```python
from build123d import *

# Parameters (mm, degrees)
SKETCH1_W           = 100
SKETCH1_H           = 55
BOSS_EXTRUDE1_DEPTH = 3
SKETCH2_W           = 100
SKETCH2_H           = 83
BOSS_EXTRUDE2_DEPTH = 3
BOSS_EXTRUDE3_DEPTH = 3
BOSS_EXTRUDE4_DEPTH = 3
SKETCH5_R           = 13
SKETCH5_R_2         = 2.15
CUT_EXTRUDE1_DEPTH  = 4


with BuildPart() as part:
    # Sketch1 → Boss-Extrude1 (new body)
    with BuildSketch(Plane(origin=(0, 0, 0), x_dir=(1, 0, 0), z_dir=(0, 1, 0))):
        Rectangle(SKETCH1_W, SKETCH1_H)
    extrude(amount=BOSS_EXTRUDE1_DEPTH)

    # Sketch2 → Boss-Extrude2 (add)
    with BuildSketch(Plane.XY.offset(27.5)):
        with Locations((0, -13.5)):
            Rectangle(SKETCH2_W, SKETCH2_H)
    extrude(amount=BOSS_EXTRUDE2_DEPTH)

    # Sketch3 → Boss-Extrude3 (add)
    with BuildSketch(Plane(origin=(50, 0, 0), x_dir=(0, 0, -1), z_dir=(1, 0, 0))):
        Polygon((-27.5, 0), (22.5, 0), (-27.5, -50), align=None)
    extrude(amount=-BOSS_EXTRUDE3_DEPTH)

    # Sketch4 → Boss-Extrude4 (add)
    with BuildSketch(Plane.ZY.offset(50)):
        Polygon((27.5, 0), (27.5, -50), (-22.5, 0), align=None)
    extrude(amount=-BOSS_EXTRUDE4_DEPTH)

    # Sketch5 → Cut-Extrude1 (cut, through all)
    with BuildSketch(Plane(origin=(0, 0, 27.5), x_dir=(-1, 0, 0), z_dir=(0, 0, -1))):
        with Locations((0, -25)):
            Circle(SKETCH5_R)
        with Locations((12.148789351, -12.404091248)):
            Circle(SKETCH5_R_2)
        with Locations((12.595908752, -37.148789351)):
            Circle(SKETCH5_R_2)
        with Locations((-12.148789351, -37.595908752)):
            Circle(SKETCH5_R_2)
        with Locations((-12.595908752, -12.851210649)):
            Circle(SKETCH5_R_2)
    extrude(amount=-CUT_EXTRUDE1_DEPTH, mode=Mode.SUBTRACT)


solid = part.part
```
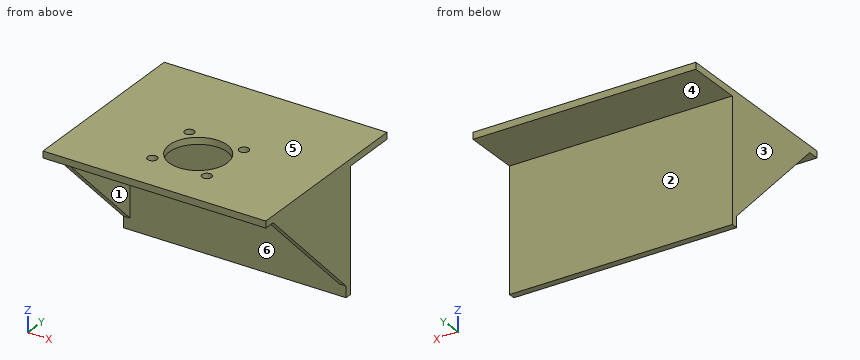
Geometry: final body of the model. Coordinates: model frame, mm. Face numbers are marked on the shaded views. A direction names the side the tool comes from. Round coordinates to 2 decimals unless told otherwise and drop trailing zeros. Order: outer loops, then holes, each group sorted by start corner. A loop starts at its lowest first (then second) coordinate and runs counter-clockwise, first axis right, second up. Notation, with made-up numbers: (78.25, 60) - (128.25, 60) arc R22 cw to (128.25, 79) - close; hole circle Ø5 at (9, -19). An arc over 180 degrees is marked (long way). Write item = value, one per line. Start each with the question number.
Q1. Cut plane C-C on z = 23. Return the cut outline in (x, y), and give its area (3 significant figures).
Q2. Access query for the marked faces 4, 5 and 6. Directions: +Z, -Z, +X, -X, +Y, -Y. A direction counts if a zero-diameter tool reaches every point of the face in a straight line with its end or side. Return the directions, or none.
Q3. Pin query (flat end, axial travel): pin 1 (3 mm diameter, centred on x = 11, z = 5, fed in from -Y); pin 2 (2 mm diameter, centred on x = 29, y = -20.5, fed in from -Z); pin 3 (1 mm diameter, centred on x = 37.5, z = 18, fed in from +Y); pin 4 (25 mm diameter, centred on y = -35.5, z = 3.5, fed in from -X). Return the tip coordinate at first contact, or that it passes through.
Q4. Pull-direction query (X, two-part tool) for the marked faces 1, 2 and 3; classes: +X half, -X half, draft (parallel to the pull), parting line (faces both ways), or undercut.
Q5. Cut plane A-A on x = 0. Return the cut outline in (y, z).
Q6. Ray query, line 1 (Y direction, x = 5, z = -1); line 2 (Z direction, x = 43, y = 7.5); line 3 (X direction, y = -17, z = 11.5). Return the intervals inside material, ascending. Write a range as from..to.
Q7. Cut plane D-D on x = -40. Return the cut outline in (y, z).
Q8. Cut plane B-B on y = -25. Return the cut outline in (x, z).
Outcome:
q1.outline = (-50, -45.5) - (-47, -45.5) - (-47, 0) - (47, 0) - (47, -45.5) - (50, -45.5) - (50, 3) - (-50, 3) - close
q1.area = 573 mm^2
q2.face_4 = -Z, +X, -X, +Y
q2.face_5 = +Z, +X, -X, +Y, -Y
q2.face_6 = -Z, -Y
q3.pin_1 = 0
q3.pin_2 = 27.5
q3.pin_3 = 3
q3.pin_4 = -50
q4.face_1 = undercut
q4.face_2 = draft
q4.face_3 = -X half
q5.outline = (-55, 27.5) - (-38, 27.5) - (-38, 30.5) - (-55, 30.5) - close; (-12, 27.5) - (0, 27.5) - (0, -27.5) - (3, -27.5) - (3, 27.5) - (28, 27.5) - (28, 30.5) - (-12, 30.5) - close
q6.line_1 = 0..3
q6.line_2 = 27.5..30.5
q6.line_3 = -50..-47, 47..50
q7.outline = (-55, 27.5) - (0, 27.5) - (0, -27.5) - (3, -27.5) - (3, 27.5) - (28, 27.5) - (28, 30.5) - (-55, 30.5) - close
q8.outline = (-50, 2.5) - (-47, 2.5) - (-47, 27.5) - (-13, 27.5) - (-13, 30.5) - (-50, 30.5) - close; (13, 27.5) - (47, 27.5) - (47, 2.5) - (50, 2.5) - (50, 30.5) - (13, 30.5) - close
